from build123d import *

# Parameters (mm, degrees)
F2_R      = 12.7
F3_DEPTH  = 25.4
F3_FACE_R = 12.7
F0_R      = 50.8
F5_T      = -2.54
F6_R      = 11.43
F7_DEPTH  = 25.4


with BuildPart() as f3:
    # F2 (on offset) → F3 (new body)
    with BuildSketch(Plane.XZ.offset(50.8)):
        Circle(F2_R)
    extrude(amount=F3_DEPTH)

    # F3_face (on face) → F4 section 0
    with BuildSketch(Plane(origin=(0, -50.8, 0), x_dir=(1, 0, 0), z_dir=(0, 1, 0))):
        Circle(F3_FACE_R)
    # F0 (on Front) → F4 section 1
    with BuildSketch(Plane.XZ):
        Circle(F0_R)
    loft()

    # F5
    f5_openings = [f3.faces().sort_by_distance(p)[0] for p in [
        (0, 0, 0),
    ]]
    offset(amount=F5_T, openings=f5_openings, kind=Kind.INTERSECTION)

    # F6 (on face) → F7 (cut)
    with BuildSketch(Plane.XZ.offset(76.2)):
        Circle(F6_R)
    extrude(amount=-F7_DEPTH, mode=Mode.SUBTRACT)


solid = f3.part
Geometry check sheet. Reference: the model listing, model coordinates, mm. A direction names the side the tool comes from. Round coordinates to 2 decimals unless told otherwise and drop trailing zeros. Loops run counter-clockwise (first coordinate to the right, second up) from the corner with the lowest first, then second, coordinate; pieces in that order, holes last. Notation, with made-up numbers: (64, 9) -> (69, 9) arc R16 ccw to (69, 18) -> close; hole circle Ø5 at (47.5, 78.25). An arc over 180 degrees is marked (long way). Answer as a JSON object with one key per item and string values. Group by question number.
Item 1: Set-up check for faces 1 (the face through (15.897, -41.278, -5.006)), 2 (the face through (-2.75, -63.32, -12.4)): record each of +Z, -Z, +X, -X, +Y, -Y from which the full face is reachable in a straight line by a thin tool's end or side.
Item 2: Release check for a two-part mould opening along X. For faces 3 (the face through (-1.323, -50.371, 10.074)), 4 (the face through (18.425, -41.978, -5.802)), 5 (the face through (-15.3, 0, 45.4)) record: pulls with the +X half, pulls with the -X half, needs draft (parallel to the pull), parting line crosses it, or undercut.
Item 3: Cross-section at C-C, the plane y = -47. Record the cut outline in (x, z) (3 decimals), plus the area to 3 significant figures.
Item 4: Depth check by flat-ended pin: pin 1 Ø4 at (x, z) = (24, 36) entering from -Y; pin 2 Ø6 at (y, z) = (-44.5, -14) entering from -X; pin 3 Ø2 at (x, z) = (-21, -3) entering from +Y. Enter the tip coordinate at first touch or a pass-through.
Item 5: Cross-section at A-A, the plane x = 0. Record the cut outline in (y, z) (3 decimals).
Item 6: Cross-section at B-B, the plane y = -36. Record the cut outline in (x, z) (3 decimals).
Item 7: Thickness scan on line 1 along Z through (x, y) = (0, -68); line 2 along X through (y, z) = (-66.5, -3); line 3 along X through (y, z) = (-50.5, 0) (3 decimals). Record the ranges inside material, lowest first.
Determined:
{
 "1": {"face 1": "+Y", "face 2": "-Y"},
 "2": {"face 3": "undercut", "face 4": "parting line crosses it", "face 5": "needs draft"},
 "3": {"outline": "circle Ø31.1 at (0, 0); hole circle Ø24.75 at (0, 0)", "area": "279 mm²"},
 "4": {"pin 1": "stops at y = -12.71", "pin 2": "stops at x = -14.86", "pin 3": "stops at y = -33.88"},
 "5": {"outline": "(-76.2, -12.7) -> (-50.8, -12.7) -> (0, -50.8) -> (0, -47.625) -> (-49.953, -10.16) -> (-50.8, -10.16) -> (-50.8, -11.43) -> (-76.2, -11.43) -> close; (-76.2, 11.43) -> (-50.8, 11.43) -> (-50.8, 10.16) -> (-49.953, 10.16) -> (0, 47.625) -> (0, 50.8) -> (-50.8, 12.7) -> (-76.2, 12.7) -> close"},
 "6": {"outline": "circle Ø47.6 at (0, 0); hole circle Ø41.25 at (0, 0)"},
 "7": {"line 1": "z = -12.7 to -11.43, 11.43 to 12.7", "line 2": "x = -12.34 to -11.03, 11.03 to 12.34", "line 3": "x = -12.925 to -10.16, 10.16 to 12.925"}
}
